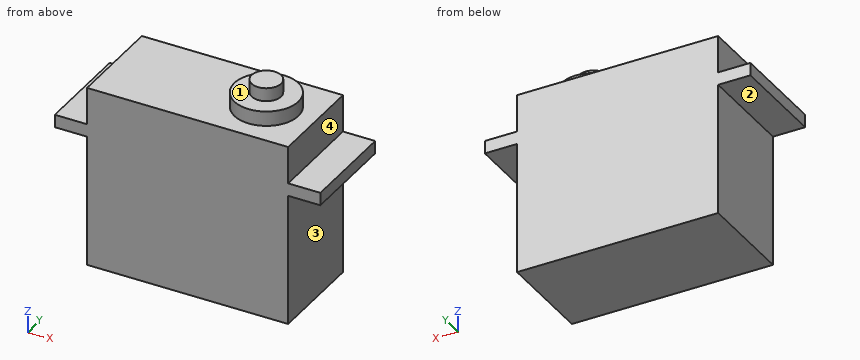
```python
from build123d import *

# Parameters (mm, degrees)
CASE_40P9_X_20_X_37_START             = -28.5
CASE_40P9_X_20_X_37_PROFILE_W         = 40.9
CASE_40P9_X_20_X_37_PROFILE_H         = 20
CASE_40P9_X_20_X_37_DEPTH             = 37
MOUNTING_TABS_54_X_20_X_2P6_START     = -1.7
MOUNTING_TABS_54_X_20_X_2P6_PROFILE_W = 54
MOUNTING_TABS_54_X_20_X_2P6_PROFILE_H = 20
MOUNTING_TABS_54_X_20_X_2P6_DEPTH     = 2.6
OUTPUT_BOSS_D13_START                 = 8.5
OUTPUT_BOSS_D13_PROFILE_R             = 6.5
OUTPUT_BOSS_D13_DEPTH                 = 3
OUTPUT_SHAFT_ENVELOPE_D6_START        = 8.5
OUTPUT_SHAFT_ENVELOPE_D6_PROFILE_R    = 3
OUTPUT_SHAFT_ENVELOPE_D6_DEPTH        = 5.7


with BuildPart() as part:
    # Case_40p9_x_20_x_37_Profile → Case_40p9_x_20_x_37 (new body)
    with BuildSketch(Plane.XY.offset(CASE_40P9_X_20_X_37_START)):
        with Locations((2.05, 0)):
            Rectangle(CASE_40P9_X_20_X_37_PROFILE_W, CASE_40P9_X_20_X_37_PROFILE_H)
    extrude(amount=CASE_40P9_X_20_X_37_DEPTH)

    # Mounting_tabs_54_x_20_x_2p6_Profile → Mounting_tabs_54_x_20_x_2p6 (add)
    with BuildSketch(Plane.XY.offset(MOUNTING_TABS_54_X_20_X_2P6_START)):
        with Locations((2.05, 0)):
            Rectangle(MOUNTING_TABS_54_X_20_X_2P6_PROFILE_W, MOUNTING_TABS_54_X_20_X_2P6_PROFILE_H)
    extrude(amount=MOUNTING_TABS_54_X_20_X_2P6_DEPTH)

    # Output_boss_D13_Profile → Output_boss_D13 (add)
    with BuildSketch(Plane.XY.offset(OUTPUT_BOSS_D13_START)):
        with Locations((12.5, 0)):
            Circle(OUTPUT_BOSS_D13_PROFILE_R)
    extrude(amount=OUTPUT_BOSS_D13_DEPTH)

    # Output_shaft_envelope_D6_Profile → Output_shaft_envelope_D6 (add)
    with BuildSketch(Plane.XY.offset(OUTPUT_SHAFT_ENVELOPE_D6_START)):
        with Locations((12.5, 0)):
            Circle(OUTPUT_SHAFT_ENVELOPE_D6_PROFILE_R)
    extrude(amount=OUTPUT_SHAFT_ENVELOPE_D6_DEPTH)


solid = part.part
```
Model file for the job. Use its own axes, mm. Face numbers are marked on the shaded views. A direction names the side the tool comes from. Coordinates: 2 decimals unless noted, no trailing zeros. Write each loop counter-clockwise with the first axis right and the second up, starting at its lowest first coordinate (ties: lowest second). Pieces come first, ordered by that corner, then holes. Notation, with made-up numbers: (24, 73.5) - (54, 73.5) arc R21 ccw to (54, 95.5) - close; hole circle Ø5 at (-15.75, -36). An arc over 180 degrees is marked (long way). One line per item, written item: value. Start each with the question number.
1. Slice it at A-A (x = 12.5). Write the cut outline in (y, z).
2. Slice it at C-C (z = 3.5). Write the cut outline in (x, y), plus the area to 3 significant figures.
3. Flat gauge pins, fed straight in: pin 1 (3.5 mm diameter, centred on x = -21.5, y = -3, fed in from -Z); pin 2 (1 mm diameter, centred on y = -1.5, z = -4.5, fed in from -X); pin 3 (7 mm diameter, centred on x = 25, y = -1.5, fed in from -Z); pin 4 (10 mm diameter, centred on x = 22.5, y = 2.5, fed in from +Z). Where does each tip first touch, or does it go through?
4. Tool access for the marked faces 1, 2, 3 and 4: list every direction of +Z, -Z, +X, -X, +Y, -Y with a clear straight run to the whole face (end or side of a thin tool).
5. Slice it at D-D (x = -12). Write the cut outline in (y, z).
6. Slice it at B-B (y = 0). Write the cut outline in (x, z), plus the area to 3 significant figures.
7. Probe line 1 (Z direction, x = -22, y = 9); line 2 (X direction, y = 2.5, z = -5); line 3 (Z direction, x = -14.5, y = -0.5). List the from-to ranges inside material, lowest first. Write a range as from..to.
Answers below:
1. outline: (-10, -28.5) - (10, -28.5) - (10, 8.5) - (6.5, 8.5) - (6.5, 11.5) - (3, 11.5) - (3, 14.2) - (-3, 14.2) - (-3, 11.5) - (-6.5, 11.5) - (-6.5, 8.5) - (-10, 8.5) - close
2. outline: (-18.4, -10) - (22.5, -10) - (22.5, 10) - (-18.4, 10) - close
2. area: 818 mm^2
3. pin 1: stops at z = -1.7
3. pin 2: stops at x = -18.4
3. pin 3: stops at z = -28.5
3. pin 4: stops at z = 11.5
4. face 1: +Z
4. face 2: -Z, -X, +Y, -Y
4. face 3: -Z, +X, +Y, -Y
4. face 4: +Z, +X, +Y, -Y
5. outline: (-10, -28.5) - (10, -28.5) - (10, 8.5) - (-10, 8.5) - close
6. outline: (-24.95, -1.7) - (-18.4, -1.7) - (-18.4, -28.5) - (22.5, -28.5) - (22.5, -1.7) - (29.05, -1.7) - (29.05, 0.9) - (22.5, 0.9) - (22.5, 8.5) - (19, 8.5) - (19, 11.5) - (15.5, 11.5) - (15.5, 14.2) - (9.5, 14.2) - (9.5, 11.5) - (6, 11.5) - (6, 8.5) - (-18.4, 8.5) - (-18.4, 0.9) - (-24.95, 0.9) - close
6. area: 1,600 mm^2
7. line 1: z = -1.7..0.9
7. line 2: x = -18.4..22.5
7. line 3: z = -28.5..8.5
